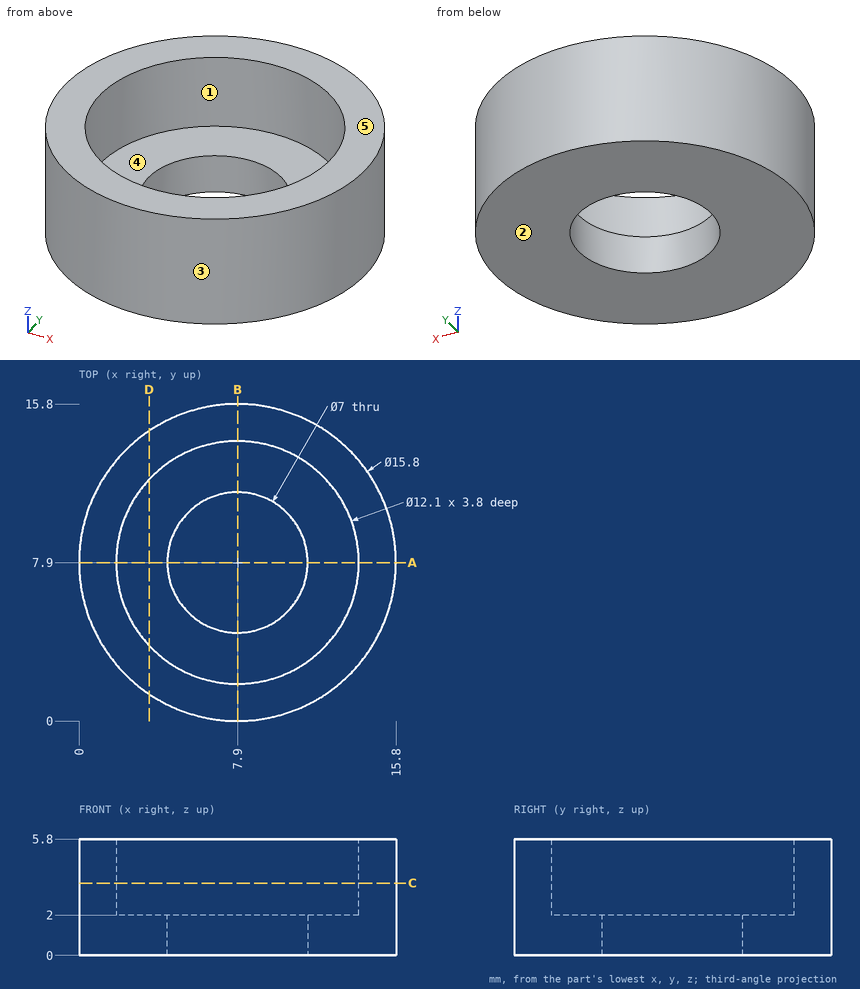
Source: three-view drawing plus pictorial views. Frame: mm from the lowest corner of the part. A direction names the side the tool comes from. Round coordinates to 2 decimals unless told otherwise and drop trailing zeros. Loops run counter-clockwise (first coordinate to the right, second up) from the corner with the lowest first, then second, coordinate; pieces in that order, holes last. Notation, with made-up numbers: M 14,7 L 48,7 A9 ccw 48,24 Z; hole C 58.25,74 d4. An arc over 180 degrees is marked long. Answer as CSV lines item,"result". Start each with the question number.
(1) Section C-C, the plane z = 3.6. Output: boundary loops of the cut face in (x, y), plus the area to 3 significant figures.
(2) Line query: line 1 (Y direction, x = 7.9, z = 0.7); line 2 (Y direction, x = 7.9, z = 4.4); line 3 (Z direction, x = 4, y = 9). Output: solid intervals per line, ascending. Write a range as [from, to].
(3) Reachability of the marked faces 1 and 2 from +Z, -Z, +X, -X, +Y, -Y: full face, straight path, thin tool, end or side. Return the list, or none.
(4) First-contact query: pin 1 (9 mm diameter, centred on x = 7.9, y = 7.9, fed in from +Z); pin 2 (3 mm diameter, centred on x = 11, z = 3, fed in from +Y); pin 3 (2 mm diameter, centred on y = 9.5, z = 5, fed in from -X). Flat tips, straight axial feed; report the tip coordinate or a pass-through.
(5) Section A-A, the plane y = 7.9. Output: boundary loops of the cut face in (x, z).
(6) Section D-D, the plane x = 3.5. Output: boundary loops of the cut face in (y, z).
(7) Draft query along X for the marked faces 3, 4 and 5. Return one class per face: released by +X, released by -X, zero draft, split by the parting line, or undercut.
Values found:
1,outline,"C 7.9,7.9 d15.8; hole C 7.9,7.9 d12.1"
1,area,"81.1 mm²"
2,line 1,"y = [0, 4.4], [11.4, 15.8]"
2,line 2,"y = [0, 1.85], [13.95, 15.8]"
2,line 3,"z = [0, 2]"
3,face 1,"+Z"
3,face 2,"-Z, +X, -X, +Y, -Y"
4,pin 1,"stops at z = 2"
4,pin 2,"stops at y = 15.64"
4,pin 3,"stops at x = 0.02"
5,outline,"M 0,0 L 4.4,0 L 4.4,2 L 1.85,2 L 1.85,5.8 L 0,5.8 Z; M 11.4,0 L 15.8,0 L 15.8,5.8 L 13.95,5.8 L 13.95,2 L 11.4,2 Z"
6,outline,"M 1.34,0 L 14.46,0 L 14.46,5.8 L 12.05,5.8 L 12.05,2 L 3.75,2 L 3.75,5.8 L 1.34,5.8 Z"
7,face 3,"split by the parting line"
7,face 4,"undercut"
7,face 5,"zero draft"
